Drawing for the job (mm, zero at the part's lowest x, y, z). A direction names the side the tool comes from. Give positions to 0.01 mm unless a question says otherwise; leave off trailing zeros. Write each loop counter-clockwise with the first axis right and the second up, starting at its lowest first coordinate (ties: lowest second). Pieces come first, ordered by that corner, then holes. Notation, with made-up numbers: (-15, 89) - (27, 89) arc R4 ccw to (27, 95) - close; hole circle Ø10 at (-36, 11). An arc over 180 degrees is marked (long way). Answer as a JSON object with one key per item and string values. Group by question number.
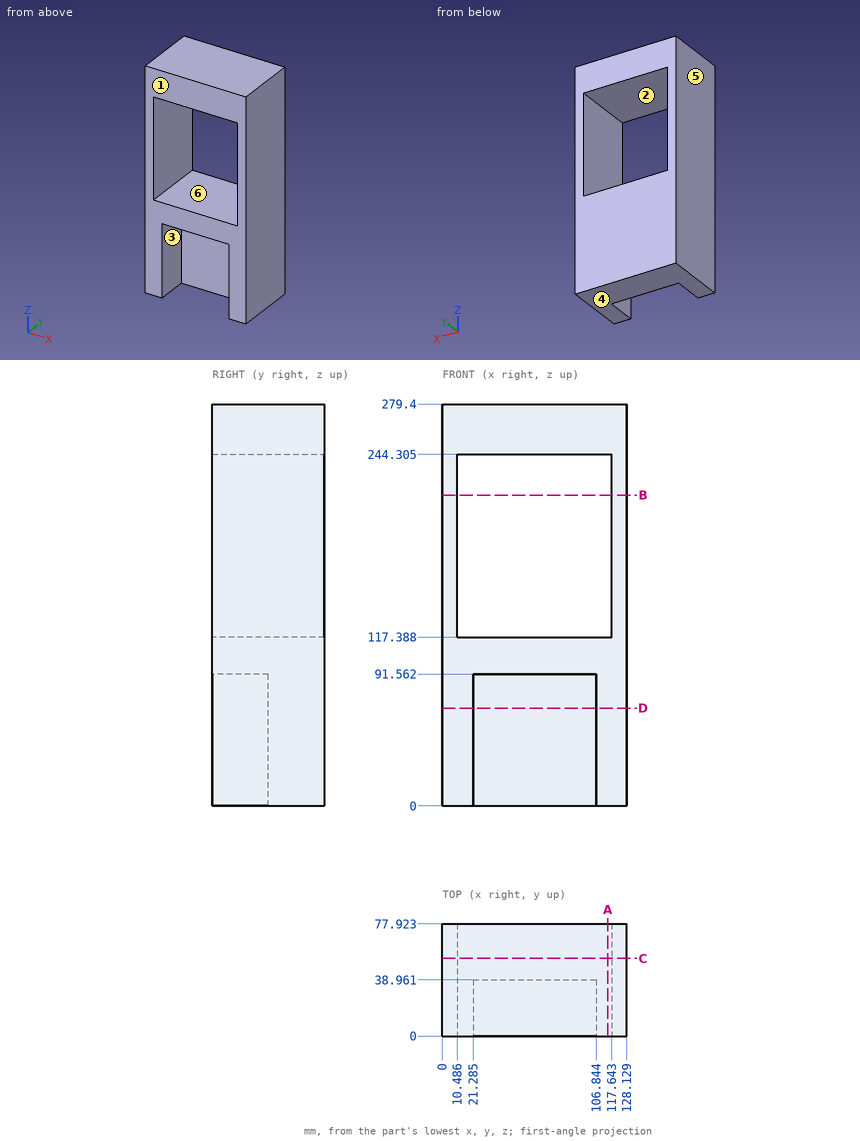
1) Band-saw the part on B-B (z = 216). List the corners of the cut face in (x, y).
2) Band-saw the part on A-A (x = 115). List the corners of the cut face in (y, z) (1 decimal).
3) Mould opens along X. For the marked faces 4, 5 and 6 say: pulls with the +X half, pulls with the -X half, needs draft (parallel to the pull), parting line crosses it, or undercut.
4) Drop flat-ended pins along their axis: P1, Ø23.5, axis at y = 29, z = 210.5, coming from the -X side; P2, Ø10, axis at x = 89.5, z = 43, coming from the -Y side; P3, Ø8, axis at x = 42.5, y = 15.5, coming from the -Z side. Give the stop position or say it passes through.
5) Band-saw the part on D-D (z = 68). List the corners of the cut face in (x, y) (1 decimal).
6) Band-saw the part on C-C (y = 54). List the corners of the cut face in (x, z) (1 decimal).
7) Which spindle directions (+Z, -Z, +X, -X, +Y, -Y) get a long thin tool onto all of the face, cutting with end or side? Do the marked faces 1, 2 and 3. Say none if no direction does.
8) Probe line 1 (X direction, y = 48, z = 231.5); line 2 (Z direction, x = 64.5, y = 54) (1 decimal); line 3 (X direction, y = 33.5, z = 44.5) (1 decimal). List the from-to ranges inside material, lowest first.
Verdict:
{
 "1": {"outline": "(0, 0) - (10.49, 0) - (10.49, 77.92) - (0, 77.92) - close; (117.64, 0) - (128.13, 0) - (128.13, 77.92) - (117.64, 77.92) - close"},
 "2": {"outline": "(0, 0) - (77.9, 0) - (77.9, 117.4) - (0, 117.4) - close; (0, 244.3) - (77.9, 244.3) - (77.9, 279.4) - (0, 279.4) - close"},
 "3": {"face 4": "needs draft", "face 5": "pulls with the -X half", "face 6": "undercut"},
 "4": {"P1": "x = 0", "P2": "y = 38.96", "P3": "z = 91.56"},
 "5": {"outline": "(0, 0) - (21.3, 0) - (21.3, 39) - (106.8, 39) - (106.8, 0) - (128.1, 0) - (128.1, 77.9) - (0, 77.9) - close"},
 "6": {"outline": "(0, 0) - (128.1, 0) - (128.1, 279.4) - (0, 279.4) - close; hole (10.5, 117.4) - (117.6, 117.4) - (117.6, 244.3) - (10.5, 244.3) - close"},
 "7": {"face 1": "+Z, -Z, +X, -X, -Y", "face 2": "+Y, -Y", "face 3": "-Z, -Y"},
 "8": {"line 1": "0 to 10.49, 117.64 to 128.13", "line 2": "0 to 117.4, 244.3 to 279.4", "line 3": "0 to 21.3, 106.8 to 128.1"}
}
